from build123d import *

# Parameters (mm, degrees)
BOSS_EXTRUDE1_DEPTH = 3
SKETCH2_R           = 1.5
CUT_EXTRUDE1_DEPTH  = 3


with BuildPart() as part:
    # Sketch1 → Boss-Extrude1 (new body)
    with BuildSketch(Plane(origin=(0, -220.619565514, 0), x_dir=(1, 0, 0), z_dir=(0, 1, 0))):
        with BuildLine():
            Line((-49.635107582, 293.830274817), (40.364892418, 293.830274817))
            ThreePointArc((40.364892418, 293.830274817), (47.435960229, 290.901342629), (50.364892418, 283.830274817))
            Line((50.364892418, 283.830274817), (50.364892418, 188.830274817))
            ThreePointArc((50.364892418, 188.830274817), (48.900426323, 185.294740911), (45.364892418, 183.830274817))
            Line((45.364892418, 183.830274817), (-54.635107582, 183.830274817))
            ThreePointArc((-54.635107582, 183.830274817), (-58.170641488, 185.294740911), (-59.635107582, 188.830274817))
            Line((-59.635107582, 188.830274817), (-59.635107582, 283.830274817))
            ThreePointArc((-59.635107582, 283.830274817), (-56.706175394, 290.901342629), (-49.635107582, 293.830274817))
        make_face()
    extrude(amount=BOSS_EXTRUDE1_DEPTH)

    # Sketch2 → Cut-Extrude1 (cut)
    with BuildSketch(Plane(origin=(0, -217.619565514, 0), x_dir=(1, 0, 0), z_dir=(0, 1, 0))):
        with Locations((-24.635107582, 290.833255232)):
            Circle(SKETCH2_R)
        with Locations((15.364892418, 290.833255232)):
            Circle(SKETCH2_R)
        with Locations((47.364892418, 272.830274817)):
            Circle(SKETCH2_R)
        with Locations((47.364892418, 211.830274817)):
            Circle(SKETCH2_R)
        with Locations((-56.635107582, 211.830274817)):
            Circle(SKETCH2_R)
        with Locations((-56.635107582, 272.830274817)):
            Circle(SKETCH2_R)
    extrude(amount=-CUT_EXTRUDE1_DEPTH, mode=Mode.SUBTRACT)


solid = part.part
Geometry: final body of the model. Coordinates: model frame, mm. Round coordinates to 2 decimals unless told otherwise and drop trailing zeros. One line per question, with ' | ' between items. Start each with the question number.
1. Contact query for a flat-ended pin moving along its axis: pin 1 (2.5 mm diameter, centred on x = 47.36, z = -272.83, fed in from -Y). Output: stop coordinate, or through.
2. Line query: line 1 along Z through (x, y) = (16.5, -218.9); line 2 along Z through (x, y) = (-52.5, -220.5); line 3 along X through (y, z) = (-218.5, -288). Output: solid intervals per line, ascending. Write a range as [from, to].
3. Mould query, pull axis Z, two halves, no side actions, for faces 1 (the face through (-4, -220.62, -240)), 2 (the face through (-5, -219, -293.83)), 3 (the face through (16.057, -219.099, -289.502)). Classes: pulls with the +Z half, pulls with the -Z half, needs draft (parallel to the pull), parting line crosses it, or undercut.
Returned:
1) pin 1: passes through
2) line 1: z = [-293.83, -291.81], [-289.85, -183.83] | line 2: z = [-293.41, -183.83] | line 3: x = [-58.72, 49.45]
3) face 1: needs draft | face 2: pulls with the -Z half | face 3: undercut
